Geometry check sheet. Reference: the model listing, model coordinates, mm. A direction names the side the tool comes from. Coordinates: 2 decimals unless noted, no trailing zeros. Loops run counter-clockwise (first coordinate to the right, second up) from the corner with the lowest first, then second, coordinate; pieces in that order, holes last.
from build123d import *

# Parameters (mm, degrees)
F0_W     = 10
F0_H     = 9
F1_DEPTH = 2.8
F3_DEPTH = 1.2
F4_W     = 2.5
F4_H     = 2.5
F5_DEPTH = 1.5
F6_R     = 2
F7_R     = 3
F8_R     = 0.6


with BuildPart() as f1:
    # F0 (on Top) → F1 (new body)
    with BuildSketch(Plane.XY):
        Rectangle(F0_W, F0_H)
    extrude(amount=F1_DEPTH)

    # F2 (on face) → F3 (join)
    with BuildSketch(Plane.XY.offset(2.8)):
        Polygon((2.15, 4.5), (-2.15, 4.5), (-2.15, 0), (-1.5, -4.5), (1.5, -4.5), (2.15, 0), align=None)
    extrude(amount=F3_DEPTH)

    # F4 (on face) → F5 (join)
    with BuildSketch(Plane(origin=(0, 0, 0), x_dir=(1, 0, 0), z_dir=(0, 0, -1))):
        with Locations((0, 1)):
            Rectangle(F4_W, F4_H)
    extrude(amount=F5_DEPTH)

    # F6
    f6_edges = [f1.edges().sort_by_distance(p)[0] for p in [
        (5, -4.5, 1.4),
        (-5, -4.5, 1.4),
    ]]
    fillet(f6_edges, radius=F6_R)

    # F7
    f7_edges = [f1.edges().sort_by_distance(p)[0] for p in [
        (0, 4.5, 4),
    ]]
    fillet(f7_edges, radius=F7_R)

    # F8
    f8_edges = [f1.edges().sort_by_distance(p)[0] for p in [
        (1.25, -2.25, -0.75),
        (-1.25, -2.25, -0.75),
        (1.25, 0.25, -0.75),
        (-1.25, 0.25, -0.75),
    ]]
    fillet(f8_edges, radius=F8_R)


solid = f1.part
(1) Sectioned sample at C-C on x = -0.5. Record the cut outline in (y, z), and give its area (3 significant figures).
Findings:
outline: (-4.5, 0) - (-2.25, 0) - (-2.25, -1.5) - (0.25, -1.5) - (0.25, 0) - (4.5, 0) - (4.5, 1) arc R3 ccw to (1.5, 4) - (-4.5, 4) - close
area: 37.8 mm2
(2) Scan lines: L1, parallel to Z at x = 3.5, y = 1.5; L2, parallel to Z at x = 0, y = -3; L3, parallel to Y at x = 1, z = 2.35. Record each from-to range of solid material in increasing order.
Findings:
L1: z = 0 to 2.8
L2: z = 0 to 4
L3: y = -4.5 to 4.18
(3) Sectioned sample at D-D on x = -2.5. Record the cut outline in (y, z), and give its area (3 significant figures).
Findings:
outline: (-4.5, 0) - (4.5, 0) - (4.5, 1) arc R3 ccw to (3.9, 2.8) - (-4.5, 2.8) - close
area: 24.9 mm2
(4) Access from +Z, -Z, +X, -X, +Y, -Y to the whole of each face (thin tool, end or side, straight path). Record for faces 1 (the flat face through (-2.15, 2, 3)), 2 (the flat face through (2.15, 1, 3)), 3 (the flat face through (0, 0.25, -1)), 4 (the flat face through (0, -2.25, -1)).
Findings:
face 1: +Z, -X, +Y, -Y
face 2: +Z, +X, +Y, -Y
face 3: -Z, +X, -X, +Y
face 4: -Z, +X, -X, -Y
(5) Gauge pin test, flat ends, axial feed: pin 1 Ø1.4 at (y, z) = (-1.5, -1) entering from +X; pin 2 Ø1 at (y, z) = (2, 3.5) entering from +X; pin 3 Ø1 at (y, z) = (-0.5, -1) entering from -X. Record the tip position at first contact, or that the pin passes through.
Findings:
pin 1: stops at x = 1.25
pin 2: stops at x = 2.15
pin 3: stops at x = -1.25
(6) Sectioned sample at B-B on y = 1. Record the cut outline in (x, z).
Findings:
outline: (-5, 0) - (5, 0) - (5, 2.8) - (2.15, 2.8) - (2.15, 4) - (-2.15, 4) - (-2.15, 2.8) - (-5, 2.8) - close
(7) Sectioned sample at A-A on z = -0.7. Record the cut outline in (x, y), and give its area (3 significant figures).
Findings:
outline: (-1.25, -1.65) arc R0.6 ccw to (-0.65, -2.25) - (0.65, -2.25) arc R0.6 ccw to (1.25, -1.65) - (1.25, -0.35) arc R0.6 ccw to (0.65, 0.25) - (-0.65, 0.25) arc R0.6 ccw to (-1.25, -0.35) - close
area: 5.94 mm2
